from build123d import *

# Parameters (mm, degrees)
BOSS_EXTRUDE1_DEPTH = 50.8
SKETCH4_W           = 5.715
SKETCH4_H           = 6.223
CUT_EXTRUDE2_DEPTH  = 51.8
FILLET1_R           = 0.381
CUT_EXTRUDE1_DEPTH  = 2.27


with BuildPart() as part:
    # Sketch2 → Boss-Extrude1 (new body)
    with BuildSketch(Plane(origin=(0, 0, 0), x_dir=(1, 0, 0), z_dir=(0, 1, 0))):
        with BuildLine():
            Line((-5.969, 0), (19.431, 0))
            ThreePointArc((19.431, 0), (19.700407684, -0.111592316), (19.812, -0.381))
            Line((19.812, -0.381), (19.812, -0.889))
            ThreePointArc((19.812, -0.889), (19.700407684, -1.158407684), (19.431, -1.27))
            Line((19.431, -1.27), (1.016, -1.27))
            ThreePointArc((1.016, -1.27), (0.746592316, -1.381592316), (0.635, -1.651))
            Line((0.635, -1.651), (0.635, -3.937))
            ThreePointArc((0.635, -3.937), (0.746592316, -4.206407684), (1.016, -4.318))
            Line((1.016, -4.318), (1.40496875, -4.318))
            ThreePointArc((1.40496875, -4.318), (1.539672592, -4.293392866), (1.656976563, -4.22275))
            ThreePointArc((1.656976563, -4.22275), (3.556, -5.08), (1.656976563, -5.93725))
            ThreePointArc((1.656976563, -5.93725), (1.539672592, -5.866607134), (1.40496875, -5.842))
            Line((1.40496875, -5.842), (-1.40496875, -5.842))
            ThreePointArc((-1.40496875, -5.842), (-1.539672592, -5.866607134), (-1.656976563, -5.93725))
            ThreePointArc((-1.656976563, -5.93725), (-3.556, -5.08), (-1.656976563, -4.22275))
            ThreePointArc((-1.656976563, -4.22275), (-1.539672592, -4.293392866), (-1.40496875, -4.318))
            Line((-1.40496875, -4.318), (-1.016, -4.318))
            ThreePointArc((-1.016, -4.318), (-0.746592316, -4.206407684), (-0.635, -3.937))
            Line((-0.635, -3.937), (-0.635, -1.651))
            ThreePointArc((-0.635, -1.651), (-0.746592316, -1.381592316), (-1.016, -1.27))
            Line((-1.016, -1.27), (-5.969, -1.27))
            ThreePointArc((-5.969, -1.27), (-6.238407684, -1.158407684), (-6.35, -0.889))
            Line((-6.35, -0.889), (-6.35, -0.381))
            ThreePointArc((-6.35, -0.381), (-6.238407684, -0.111592316), (-5.969, 0))
        make_face()
    extrude(amount=BOSS_EXTRUDE1_DEPTH)

    # Sketch4 → Cut-Extrude2 (cut, through all)
    with BuildSketch(Plane.XZ):
        with Locations((-3.4925, 3.1115)):
            Rectangle(SKETCH4_W, SKETCH4_H)
    extrude(amount=-CUT_EXTRUDE2_DEPTH, mode=Mode.SUBTRACT)

    # Fillet1
    fillet1_edges = [part.edges().sort_by_distance(p)[0] for p in [
        (-0.635, 25.4, 5.842),
        (-0.635, 25.4, 0),
    ]]
    fillet(fillet1_edges, radius=FILLET1_R)

    # Sketch3 → Cut-Extrude1 (cut, through all)
    with BuildSketch(Plane.XY.offset(1.27)):
        with BuildLine():
            Line((8.2931, 27.3812), (9.8806, 27.3812))
            Line((9.8806, 27.3812), (9.8806, 28.9814))
            ThreePointArc((9.8806, 28.9814), (11.8618, 30.9626), (13.843, 28.9814))
            Line((13.843, 28.9814), (13.843, 27.3812))
            Line((13.843, 27.3812), (15.4305, 27.3812))
            ThreePointArc((15.4305, 27.3812), (17.4117, 25.4), (15.4305, 23.4188))
            Line((15.4305, 23.4188), (8.2931, 23.4188))
            ThreePointArc((8.2931, 23.4188), (6.3119, 25.4), (8.2931, 27.3812))
        make_face()
    extrude(amount=-CUT_EXTRUDE1_DEPTH, mode=Mode.SUBTRACT)


solid = part.part
Work out the finished part from the listing and answer in its coordinate system (mm). A direction names the side the tool comes from. Coordinates: 2 decimals unless noted, no trailing zeros. Write each loop counter-clockwise with the first axis right and the second up, starting at its lowest first coordinate (ties: lowest second). Pieces come first, ordered by that corner, then holes. Notation, with made-up numbers: M -19.75,-25 L -13.75,-25 A28 cw -13.75,5 Z; hole C 67,-10.5 d2. An arc over 180 degrees is marked long. Use one line per item in the form item = value. Start each with the question number.
1. The mould has two halves that part along Y. Classify faces 4 (the face through (7, 50.8, 1)), 5 (the face through (6, 25, 1.27)), 6 (the face through (12, 23.419, 1)), 7 (the face through (7, 0, 1)): released by +Y, released by -Y, zero draft, split by the parting line, or undercut.
2. Straight lines are drawn through the part: probe 1 along Z at (x, y) = (1.25, 4.5); probe 2 along Z at (x, y) = (2.5, 30.5); probe 3 along Z at (x, y) = (8.5, 8). For each, find the intervals that lie inside material, in ascending order. Write a range as from..to.
3. Each of these flat-tipped pins is pushed along its axis until it touches: P1, Ø0.5, axis at x = 1, y = 29.5, coming from the +Z side; P2, Ø1, axis at y = 21, z = 5, coming from the +X side; P3, Ø1.1, axis at y = 22, z = 2.5, coming from the +X side (3 decimals). Where does it stop, or does it pass through?
4. The part is cut by section B-B (x = 16). Give the vertices of the cut face in (y, z), plus the area to 3 significant figures.
5. The part is cut by section C-C (y = 45.5). Give the vertices of the cut face in (x, z) (3 decimals).
6. A tool of negligible diameter and unlimited length cuts with its end or side. For faces 1 (the face through (9.881, 28, 1)), 2 (the face through (0.635, 25, 3)), 3 (the face through (1, 25, 5.842)), from which of +Z, -Z, +X, -X, +Y, -Y can it reach the whole face along a straight path? Write none if from no direction.
7. The part is cut by section D-D (x = 7.75). Give the vertices of the cut face in (y, z), plus the area to 3 significant figures.
8. The part is cut by section A-A (y = 25.4). Give the vertices of the cut face in (x, z) (3 decimals), plus the area to 3 significant figures.
Evaluation:
q1.face_4 = released by +Y
q1.face_5 = zero draft
q1.face_6 = undercut
q1.face_7 = released by -Y
q2.probe_1 = 0..1.27, 4.32..5.84
q2.probe_2 = 0..1.27, 3.94..6.22
q2.probe_3 = 0..1.27
q3.P1 = 5.84
q3.P2 = 3.56
q3.P3 = 0.635
q4.outline = M 0,0 L 23.5,0 L 23.5,1.27 L 0,1.27 Z; M 27.3,0 L 50.8,0 L 50.8,1.27 L 27.3,1.27 Z
q4.area = 59.7 mm^2
q5.outline = M -0.635,0.381 A0.381 ccw -0.254,0 L 19.431,0 A0.381 ccw 19.812,0.381 L 19.812,0.889 A0.381 ccw 19.431,1.27 L 1.016,1.27 A0.381 cw 0.635,1.651 L 0.635,3.937 A0.381 cw 1.016,4.318 L 1.405,4.318 A0.381 cw 1.657,4.223 A1.143 ccw long 1.657,5.937 A0.381 cw 1.405,5.842 L -0.254,5.842 A0.381 ccw -0.635,5.461 Z
q6.face_1 = +Z, -Z
q6.face_2 = +X, +Y, -Y
q6.face_3 = +Z, -X, +Y, -Y
q7.outline = M 0,0 L 23.49,0 L 23.49,1.27 L 0,1.27 Z; M 27.31,0 L 50.8,0 L 50.8,1.27 L 27.31,1.27 Z
q7.area = 59.7 mm^2
q8.outline = M -0.635,0.381 A0.381 ccw -0.254,0 L 6.312,0 L 6.312,1.27 L 1.016,1.27 A0.381 cw 0.635,1.651 L 0.635,3.937 A0.381 cw 1.016,4.318 L 1.405,4.318 A0.381 cw 1.657,4.223 A1.143 ccw long 1.657,5.937 A0.381 cw 1.405,5.842 L -0.254,5.842 A0.381 ccw -0.635,5.461 Z; M 17.412,0 L 19.431,0 A0.381 ccw 19.812,0.381 L 19.812,0.889 A0.381 ccw 19.431,1.27 L 17.412,1.27 Z
q8.area = 22.8 mm^2
